Part model, mm, in its own coordinate system. A direction names the side the tool comes from. Round coordinates to 2 decimals unless told otherwise and drop trailing zeros. Order: outer loops, then holes, each group sorted by start corner. A loop starts at its lowest first (then second) coordinate and runs counter-clockwise, first axis right, second up. Notation, with made-up numbers: (33.5, 33) - (37.5, 33) arc R29 ccw to (37.5, 72) - close; hole circle Ø3 at (-17.75, 48.5). An arc over 180 degrees is marked (long way). Answer as a JSON object with one key per item and string values.
```python
from build123d import *

# Parameters (mm, degrees)
F0_W     = 127
F0_H     = 76.2
F1_DEPTH = 63.5
F2_W     = 76.2
F2_H     = 50.8
F3_DEPTH = 63.5
F4_R     = 50.8
F5_DEPTH = 132.08
F6_W     = 25.4
F6_H     = 25.4
F7_DEPTH = 25.4


with BuildPart() as f1:
    # F0 (on Front) → F1 (new body)
    with BuildSketch(Plane.XZ):
        Rectangle(F0_W, F0_H)
    extrude(amount=F1_DEPTH)

    # F2 (on face) → F3 (cut)
    with BuildSketch(Plane.XZ.offset(63.5)):
        with Locations((0, 12.7)):
            Rectangle(F2_W, F2_H)
    extrude(amount=-F3_DEPTH, mode=Mode.SUBTRACT)

    # F4 (on face) → F5 (cut)
    with BuildSketch(Plane(origin=(-63.5, 0, 0), x_dir=(0, -1, 0), z_dir=(-1, 0, 0))):
        with Locations((63.5, 38.1)):
            Circle(F4_R)
    extrude(amount=-F5_DEPTH, mode=Mode.SUBTRACT)

    # F6 (on face) → F7 (cut)
    with BuildSketch(Plane.XY.offset(-12.7)):
        with Locations((0, -38.1)):
            Rectangle(F6_W, F6_H)
    extrude(amount=-F7_DEPTH, mode=Mode.SUBTRACT)


solid = f1.part
```
Item 1: Tool access for faces 4 (the cylindrical face through (-50.978, -27.186, 2.576)), 5 (the flat face through (-12.7, -38, -25)), 6 (the flat face through (-38.1, -18, 7)): list every direction of +Z, -Z, +X, -X, +Y, -Y with a clear straight run to the whole face (end or side of a thin tool).
Taken from the geometry:
{"face 4": "+Z, +X, -X, -Y", "face 5": "+Z, -Z", "face 6": "+Z, +Y, -Y"}
Item 2: Two-plate mould, pull along X, no slides. Class faces 1 (the flat face through (38.1, -18, 7)), 2 (the flat face through (51, -6, 38.1)), 3 (the flat face through (-63.5, -24, -9)): pulls with the +X half, pulls with the -X half, needs draft (parallel to the pull), parting line crosses it, or undercut.
Taken from the geometry:
{"face 1": "undercut", "face 2": "needs draft", "face 3": "pulls with the -X half"}
Item 3: Cut at A-A (x = -5.5). Write the cut outline in (y, z).
Taken from the geometry:
{"outline": "(-63.5, -38.1) - (-50.8, -38.1) - (-50.8, -12.7) - (-63.5, -12.7) - close; (-25.4, -38.1) - (0, -38.1) - (0, -12.7) - (-25.4, -12.7) - close"}
Item 4: Cut at C-C (y = -29.5). Write the cut outline in (x, z).
Taken from the geometry:
{"outline": "(-63.5, -38.1) - (-12.7, -38.1) - (-12.7, -12.7) - (-38.1, -12.7) - (-38.1, 0.36) - (-63.5, 0.36) - close; (12.7, -38.1) - (63.5, -38.1) - (63.5, 0.36) - (38.1, 0.36) - (38.1, -12.7) - (12.7, -12.7) - close"}
Item 5: Cut at D-D (z = 5). Write the cut outline in (x, y), plus the area to 3 significant figures.
Taken from the geometry:
{"outline": "(-63.5, -24.96) - (-38.1, -24.96) - (-38.1, 0) - (-63.5, 0) - close; (38.1, -24.96) - (63.5, -24.96) - (63.5, 0) - (38.1, 0) - close", "area": "1,270 mm2"}
Item 6: Probe L1, parallel to Y at x = -0.5, z = -13; L2, parallel to X at y = -12, z = -10; L3, parallel to X at y = -27.5, z = -27. List the from-to ranges inside material, lowest first. Write a range as from..to.
Taken from the geometry:
{"L1": "-63.5..-50.8, -25.4..0", "L2": "-63.5..-38.1, 38.1..63.5", "L3": "-63.5..-12.7, 12.7..63.5"}
Item 7: Drop a flat-ended pin along its axis: P1, Ø6, axis at x = 20, y = -49.5, coming from the +Z side. Give the stop position or say it passes through.
Taken from the geometry:
{"P1": "z = -12.7"}
Item 8: Cut at B-B (z = -25.5). Write the cut outline in (x, y), plus the area to 3 significant figures.
Taken from the geometry:
{"outline": "(-63.5, -63.5) - (63.5, -63.5) - (63.5, 0) - (-63.5, 0) - close; hole (-12.7, -50.8) - (12.7, -50.8) - (12.7, -25.4) - (-12.7, -25.4) - close", "area": "7,420 mm2"}
